Read the model definition and answer for the solid it produces. Units are mm, in the model's axes. A direction names the side the tool comes from. Coordinates: 2 decimals unless noted, no trailing zeros. Order: outer loops, then holes, each group sorted by start corner. A loop starts at its lowest first (then second) coordinate and runs counter-clockwise, first axis right, second up.
```python
from build123d import *

# Parameters (mm, degrees)
SKETCH1_W           = 105
SKETCH1_H           = 100
SKETCH1_R           = 2.5
BOSS_EXTRUDE2_DEPTH = 16
SKETCH2_R           = 45
CUT_EXTRUDE1_DEPTH  = 12
CHAMFER1_SIZE       = 5


with BuildPart() as part:
    # Sketch1 → Boss-Extrude2 (new body)
    with BuildSketch(Plane(origin=(0, 0, 0), x_dir=(1, 0, 0), z_dir=(0, 1, 0))):
        Rectangle(SKETCH1_W, SKETCH1_H)
        with Locations((47, -37)):
            Circle(SKETCH1_R, mode=Mode.SUBTRACT)
        with Locations((47, 37)):
            Circle(SKETCH1_R, mode=Mode.SUBTRACT)
        with Locations((-47, 37)):
            Circle(SKETCH1_R, mode=Mode.SUBTRACT)
        with Locations((-47, -37)):
            Circle(SKETCH1_R, mode=Mode.SUBTRACT)
    extrude(amount=BOSS_EXTRUDE2_DEPTH)

    # Sketch2 → Cut-Extrude1 (cut)
    with BuildSketch(Plane(origin=(0, 0, 0), x_dir=(1, 0, 0), z_dir=(0, 1, 0))):
        Circle(SKETCH2_R)
    extrude(amount=CUT_EXTRUDE1_DEPTH, mode=Mode.SUBTRACT)

    # Chamfer1
    chamfer1_edges = [part.edges().sort_by_distance(p)[0] for p in [
        (-45, 12, 0),
    ]]
    chamfer(chamfer1_edges, length=CHAMFER1_SIZE)


solid = part.part
```
1) A cutting plane is placed at D-D, the plane z = -37. State how many separate pieces and enclosed holes the cut face has, and give its area (3 significant figures).
A:
separate pieces: 3
enclosed holes: 0
area: 954 mm2
2) Determine the mould class of faces 3 (the cylindrical face through (49.31, 7.89, 37.96)), 4 (the flat face through (-52.5, 8, 1)), 5 (the flat face through (-1, 8, -50)), 6 (the flat face through (52.5, 8, 1)) for opening direction X: pulls with the +X half, pulls with the -X half, needs draft (parallel to the pull), parting line crosses it, or undercut.
A:
face 3: undercut
face 4: pulls with the -X half
face 5: needs draft
face 6: pulls with the +X half
3) A cutting plane is placed at B-B, the plane y = 5.25. Determine the outline of the cut face in (x, z), and give its area (3 significant figures).
A:
outline: (-52.5, -50) - (52.5, -50) - (52.5, 50) - (-52.5, 50) - close; hole circle Ø5 at (-47, -37); hole circle Ø5 at (-47, 37); hole circle Ø90 at (0, 0); hole circle Ø5 at (47, -37); hole circle Ø5 at (47, 37)
area: 4,060 mm2
4) A cutting plane is placed at A-A, the plane x = -47. Determine the outline of the cut face in (y, z), and give its area (3 significant figures).
A:
outline: (0, -50) - (16, -50) - (16, -39.5) - (0, -39.5) - close; (0, -34.5) - (16, -34.5) - (16, 34.5) - (0, 34.5) - close; (0, 39.5) - (16, 39.5) - (16, 50) - (0, 50) - close
area: 1,440 mm2
5) Which of the six approach directions +Z, -Z, +X, -X, +Y, -Y give full straight-line access (tool end or side, diameter ignored) to faces 1 (the flat face through (-1, 12, -1)), 2 (the cylindrical face through (-44.69, 7.89, -36.04))?
A:
face 1: -Y
face 2: +Y, -Y
6) A cutting plane is placed at C-C, the plane x = 0. Determine the outline of the cut face in (y, z), and give its area (3 significant figures).
A:
outline: (0, -50) - (16, -50) - (16, 50) - (0, 50) - (0, 45) - (7, 45) - (12, 40) - (12, -40) - (7, -45) - (0, -45) - close
area: 545 mm2
7) Straight lines are drawn through the part: line 1 (Z direction, x = 47, y = 10); line 2 (X direction, y = 12.75, z = 37); line 3 (Y direction, x = 0.5, z = 3.5). For each, find the intervals that lie inside material, in ascending order.
A:
line 1: z = -50 to -39.5, -34.5 to 34.5, 39.5 to 50
line 2: x = -52.5 to -49.5, -44.5 to 44.5, 49.5 to 52.5
line 3: y = 12 to 16
8) Flat-ended cylindrical pins translate along their axes: pin 1 Ø4 at (x, z) = (-47, -37) entering from +Y; pin 2 Ø10 at (x, z) = (19, -0.5) entering from -Y. Find the tip coordinate at first contact, or state that the pin passes through.
A:
pin 1: passes through
pin 2: stops at y = 12
